Model file for the job. Use its own axes, mm. Face numbers are marked on the shaded views. A direction names the side the tool comes from. Coordinates: 2 decimals unless noted, no trailing zeros. Write each loop counter-clockwise with the first axis right and the second up, starting at its lowest first coordinate (ties: lowest second). Pieces come first, ordered by that corner, then holes. Notation, with made-up numbers: M 6.25,14 L 35.25,14 A18 ccw 35.25,47 Z; hole C -29,-11.5 d3. An arc over 180 degrees is marked long. One line per question, with ' | ' between items. Start each with the question number.
(1) Two-plate mould, pull along Y, no slides. Class the marked faces 3, 4 and 5: +Y half, -Y half, draft (parallel to the pull), parting line (faces both ways), or undercut.
(2) Cut at C-C (x = 1.6). Write the cut outline in (y, z).
(3) Flat gauge pins, fed straight in: pin 1 Ø1.5 at (x, z) = (-2, -2.5) entering from -Y; pin 2 Ø2 at (x, y) = (0, 0) entering from +Z; pin 3 Ø1 at (y, z) = (-2.5, 1.5) entering from -X. Where does each tip first touch, or does it go through?
(4) Cut at D-D (z = -2). Write the cut outline in (x, y), plus the area to 3 significant figures.
(5) Wall check: probe 1 along Y at (x, z) = (0, 6.9); probe 2 along X at (y, z) = (0.7, -8); probe 3 along Y at (x, z) = (0.65, -4.5). Give the ranges that are in metal, low to high.
(6) Cut at A-A (z = 6.5). Write the cut outline in (x, y).
(7) Tool access for the marked faces 1 and 2: list every direction of +Z, -Z, +X, -X, +Y, -Y with a clear straight run to the whole face (end or side of a thin tool).
(8) Cut at B-B (y = -1.8). Write the cut outline in (x, z).
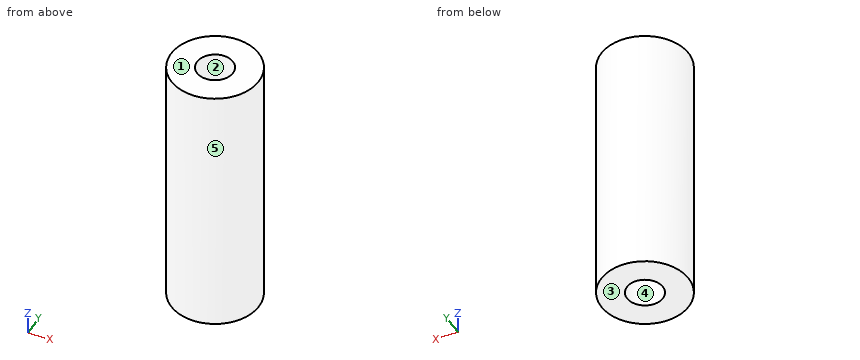
Autodesk Inventor part; units mm, degrees
ref_plane "YZ Plane" through (0, 0, 0) normal (1, 0, 0) x (0, 1, 0)
ref_plane "XZ Plane" through (0, 0, 0) normal (0, 1, 0) x (-1, 0, 0)
ref_plane "XY Plane" through (0, 0, 0) normal (0, 0, 1) x (1, 0, 0)
sketch "Skizze1" plane through (0, 0, 0) normal (0, 0, 1) x (1, 0, 0)
  circle A0 centre (0, 0) radius 3
  dimension "d0" = 6
extrude "Extrusion1" add sketch "Skizze1" along normal mid plane 18
sketch "Skizze3" plane through (0, 0, -9) normal (0, 0, -1) x (-1, 0, 0)
  point P0 (0, 0)
  point P1 (0, 0)
hole "Bohrung2" at (0, 0, -9) direction (0, 0, 1) diameter 2.459 depth 6 tip angle 118
mirror "Spiegeln1" about plane through (0, 0, 0) normal (0, 0, 1) of "Bohrung2"
properties part number "Abstandsbolzen_Kamera"
Filled in:
1) face 3: draft | face 4: undercut | face 5: parting line
2) outline: M -2.54,-9 L 2.54,-9 L 2.54,9 L -2.54,9 Z
3) pin 1: y = -2.73 | pin 2: z = 2.86 | pin 3: x = -2.24
4) outline: C 0,0 d6 | area: 28.3 mm²
5) probe 1: -3 to -1.23, 1.23 to 3 | probe 2: -2.92 to -1.01, 1.01 to 2.92 | probe 3: -2.93 to -1.04, 1.04 to 2.93
6) outline: C 0,0 d6; hole C 0,0 d2.46
7) face 1: +Z, +X, -X, +Y, -Y | face 2: +Z
8) outline: M -2.4,-9 L 2.4,-9 L 2.4,9 L -2.4,9 Z
